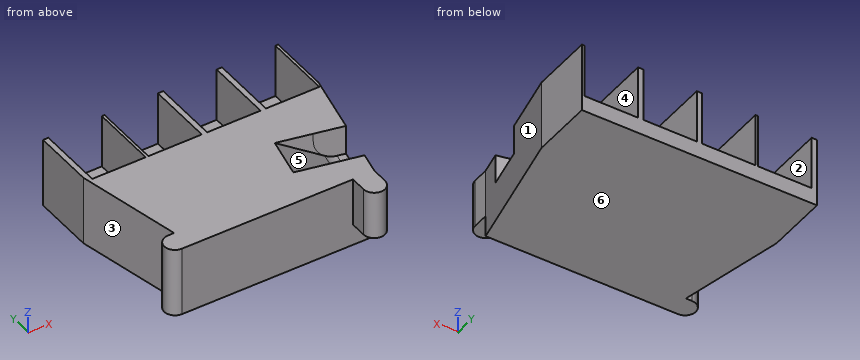
```python
from build123d import *

# Parameters (mm, degrees)
EXTRUDE_1_DEPTH      = 26
SKETCH_4_W           = 20
SKETCH_4_H           = 20
CUT_EXTRUDE_5_DEPTH  = 25
CUT_EXTRUDE_6_DEPTH  = 8
CUT_EXTRUDE_8_DEPTH  = 16
SKETCH_12_W          = 8
SKETCH_12_H          = 10
EXTRUDE_2_DEPTH      = 26
CUT_EXTRUDE_9_DEPTH  = 26
SKETCH_14_W          = 8
SKETCH_14_H          = 12.86312638
CUT_EXTRUDE_10_DEPTH = 95.212525707


with BuildPart() as part:
    # 草图1 → 凸台-拉伸1 (new body)
    with BuildSketch(Plane.XY):
        Polygon((-34, -24), (34, -24), (44, 23), (44, 46), (-44, 46), (-44, 23), align=None)
    extrude(amount=EXTRUDE_1_DEPTH)

    # 草图4 → 切除-拉伸5 (cut)
    with BuildSketch(Plane(origin=(0, 46, 0), x_dir=(1, 0, 0), z_dir=(0, 1, 0))):
        with Locations((33, -16)):
            Rectangle(SKETCH_4_W, SKETCH_4_H)
        with Locations((11, -16)):
            Rectangle(SKETCH_4_W, SKETCH_4_H)
        with Locations((-11, -16)):
            Rectangle(SKETCH_4_W, SKETCH_4_H)
        with Locations((-32, -16)):
            Rectangle(SKETCH_4_W, SKETCH_4_H)
    extrude(amount=-CUT_EXTRUDE_5_DEPTH, mode=Mode.SUBTRACT)

    # Sketch 3D_6 → 切除-拉伸6 (cut, symmetric)
    with BuildSketch(Plane(origin=(34.478414998, -7.335832978, 14.99907516), x_dir=(0.5895982688198705, -0.12544644017993214, 0.7978954016979886), z_dir=(-0.20810764446495697, -0.9781059289848145, -6.6559639472978385e-12))):
        with BuildLine():
            Line((0, 0), (6.376045072, -8.439700449))
            Line((6.376045072, -8.439700449), (17.547318622, 0))
            Line((17.547318622, 0), (11.17127355, 8.439700449))
            Line((11.17127355, 8.439700449), (6.348906145, 14.822863662))
            Line((6.348906145, 14.822863662), (1.560795809, 11.205530619))
            ThreePointArc((1.560795809, 11.205530619), (-1.540343474, 5.926016705), (0, 0))
        make_face()
    extrude(amount=CUT_EXTRUDE_6_DEPTH, both=True, mode=Mode.SUBTRACT)

    # 草图11 → 切除-拉伸8 (cut)
    with BuildSketch(Plane(origin=(-1.664861156, -7.824847432, 0), x_dir=(0.9781059289845859, -0.2081076444660318, -1.1269708570671002e-12), z_dir=(0.20810764446603178, 0.9781059289845858, 5.296763028184159e-12))):
        with BuildLine():
            Line((31.200844283, -16.100518909), (14.333584528, -26))
            Line((14.333584528, -26), (32.666556858, -30.571318601))
            ThreePointArc((32.666556858, -30.571318601), (42.196349228, -26.968728166), (40.460809076, -16.92962956))
            Line((40.460809076, -16.92962956), (38.250185053, -14.99907516))
            Line((38.250185053, -14.99907516), (35.250185053, -15))
            ThreePointArc((35.250185053, -15), (33.152072655, -15.280030806), (31.200844283, -16.100518909))
        make_face()
    extrude(amount=CUT_EXTRUDE_8_DEPTH, mode=Mode.SUBTRACT)

    # 草图12 → 凸台-拉伸2 (add)
    with BuildSketch(Plane(origin=(0, 0, 0), x_dir=(-1, 0, 0), z_dir=(0, 0, -1))):
        with Locations((-30, -29)):
            Rectangle(SKETCH_12_W, SKETCH_12_H)
        with BuildLine():
            Line((34, -24), (38, -24))
            ThreePointArc((38, -24), (42, -20), (38, -16))
            Line((38, -16), (34, -16))
            Line((34, -16), (34, -24))
        make_face()
    extrude(amount=-EXTRUDE_2_DEPTH)

    # 草图13 → 切除-拉伸9 (cut)
    with BuildSketch(Plane(origin=(0, 0, 0), x_dir=(-1, 0, 0), z_dir=(0, 0, -1))):
        with BuildLine():
            Line((-34, -30), (-34, -35.772176756))
            Line((-34, -35.772176756), (-26, -35.772176756))
            Line((-26, -35.772176756), (-26, -30))
            ThreePointArc((-26, -30), (-30, -34), (-34, -30))
        make_face()
        with BuildLine():
            Line((26, -30), (26, -35.772176756))
            Line((26, -35.772176756), (34, -35.772176756))
            Line((34, -35.772176756), (34, -30))
            ThreePointArc((34, -30), (30, -34), (26, -30))
        make_face()
    extrude(amount=-CUT_EXTRUDE_9_DEPTH, mode=Mode.SUBTRACT)

    # 草图14 → 切除-拉伸10 (cut, through all)
    with BuildSketch(Plane(origin=(34, 0, 0), x_dir=(0, 0, -1), z_dir=(1, 0, 0))):
        with Locations((-4, -30.43156319)):
            Rectangle(SKETCH_14_W, SKETCH_14_H)
    extrude(amount=-CUT_EXTRUDE_10_DEPTH, mode=Mode.SUBTRACT)


solid = part.part
```
Build history of the part. All positions in model axes, mm. Face numbers are marked on the shaded views. A direction names the side the tool comes from. Coordinates: 2 decimals unless noted, no trailing zeros. Order: outer loops, then holes, each group sorted by start corner. A loop starts at its lowest first (then second) coordinate and runs counter-clockwise, first axis right, second up.
Item 1: Drop flat-ended pins along their axis: pin 1 Ø10 at (x, y) = (-34, 32) entering from +Z; pin 2 Ø2.5 at (x, y) = (28.5, -31) entering from -Z; pin 3 Ø2 at (x, z) = (-30, 5.5) entering from -Y. Give the stop position or say it passes through.
Filled in:
pin 1: stops at z = 6
pin 2: stops at z = 8
pin 3: stops at y = -24
Item 2: Saw through at C-C on y = -20. List the corners of the cut face in (x, z).
Filled in:
outline: (-42, 0) - (34.85, 0) - (34.85, 26) - (-42, 26) - close
Item 3: Drill centre lines: L1, parallel to X at y = 30.5, z = 15.25; L2, parallel to Y at x = 15, z = 13.75; L3, parallel to Y at x = 0, z = 15.5. Where is each one in solid material? Low to high.
Filled in:
L1: x = -44 to -42, -22 to -21, -1 to 1, 21 to 23, 43 to 44
L2: y = -24 to 21
L3: y = -24 to 46
Item 4: Saw through at B-B on x = -29. List the corners of the cut face in (y, z).
Filled in:
outline: (-24, 0) - (46, 0) - (46, 6) - (21, 6) - (21, 26) - (-24, 26) - close
Item 5: Saw through at D-D on x = 22. List the corners of the cut face in (y, z).
Filled in:
outline: (-24, 0) - (46, 0) - (46, 26) - (3.5, 26) - (3.5, 22.21) - (-12.86, 20.21) - (-12.86, 26) - (-24, 26) - close
Item 6: Saw through at A-A on z = 4.75. List the corners of the cut face in (x, y), then the cut area to 3 significant figures.
Filled in:
outline: (-44, 23) - (-35.7, -16) - (-38, -16) arc R4 ccw to (-38, -24) - (34, -24) - (44, 23) - (44, 46) - (-44, 46) - close
area: 5,740 mm2
Item 7: Tool access for the marked faces 4, 5 and 6: list every direction of +Z, -Z, +X, -X, +Y, -Y with a clear straight run to the whole face (end or side of a thin tool).
Filled in:
face 4: +Z, +Y
face 5: +Z
face 6: -Z, +X, -X, +Y, -Y
Item 8: Mould opens along Y. For the marked faces 1, 2 and 3 say: released by +Y, released by -Y, zero draft, split by the parting line, or undercut.
Filled in:
face 1: released by -Y
face 2: zero draft
face 3: undercut
